```python
from build123d import *

# Parameters (mm, degrees)
SKETCH1_W               = 3.3
SKETCH1_H               = 7.4
BOSS_EXTRUDE1_DEPTH     = 2.6
BOSS_EXTRUDE1_2_DEPTH   = 2.6
BOSS_EXTRUDE1_3_DEPTH   = 2.6
SKETCH1_W_2             = 18
SKETCH1_H_2             = 1.6
BOSS_EXTRUDE1_4_DEPTH   = 2.6
BOSS_EXTRUDE1_5_DEPTH   = 2.6
SKETCH3_W               = 18
SKETCH3_H               = 22.9
BOSS_EXTRUDE2_DEPTH     = 1.6
CUT_EXTRUDE1_DEPTH      = 27.511924597
CUT_EXTRUDE1_DEPTH_BACK = 27.511924597
FILLET1_R               = 2
FILLET2_R               = 1


with BuildPart() as part:
    # Sketch1 → Boss-Extrude1 (new body)
    with BuildSketch(Plane.XY):
        with Locations((-6.907290918, -7.556371191)):
            Rectangle(SKETCH1_W, SKETCH1_H)
    extrude(amount=BOSS_EXTRUDE1_DEPTH)



with BuildPart() as body_2:
    # Sketch1 → Boss-Extrude1 2 (new body)
    with BuildSketch(Plane.XY):
        with Locations((0.442709082, -7.556371191)):
            Rectangle(SKETCH1_W, SKETCH1_H)
    extrude(amount=BOSS_EXTRUDE1_2_DEPTH)


with BuildPart() as body_3:
    # Sketch1 → Boss-Extrude1 3 (new body)
    with BuildSketch(Plane.XY):
        with Locations((7.792709082, -7.556371191)):
            Rectangle(SKETCH1_W, SKETCH1_H)
    extrude(amount=BOSS_EXTRUDE1_3_DEPTH)


with BuildPart() as body_4:
    # Sketch1 → Boss-Extrude1 4 (new body)
    with BuildSketch(Plane.XY):
        with Locations((0.442709082, 3.093628809)):
            Rectangle(SKETCH1_W_2, SKETCH1_H_2)
    extrude(amount=BOSS_EXTRUDE1_4_DEPTH)


with BuildPart() as body_5:
    # Sketch1 → Boss-Extrude1 5 (new body)
    with BuildSketch(Plane.XY):
        with Locations((0.442709082, -18.206371191)):
            Rectangle(SKETCH1_W_2, SKETCH1_H_2)
    extrude(amount=BOSS_EXTRUDE1_5_DEPTH)


with BuildPart() as part_1:
    add(part.part)

    add(body_2.part)  # Boss-Extrude2 merges body 2

    add(body_3.part)  # Boss-Extrude2 merges body 3

    add(body_4.part)  # Boss-Extrude2 merges body 4

    add(body_5.part)  # Boss-Extrude2 merges body 5
    # Sketch3 → Boss-Extrude2 (add)
    with BuildSketch(Plane.XY.offset(2.6)):
        with Locations((0.442709082, -7.556371191)):
            Rectangle(SKETCH3_W, SKETCH3_H)
    extrude(amount=BOSS_EXTRUDE2_DEPTH)

    # Sketch4 → Cut-Extrude1 (cut, two sides: drawn at the far end of the back side and taken through both)
    with BuildSketch(Plane.ZY.offset(8.557290918).offset(-CUT_EXTRUDE1_DEPTH_BACK)):
        Polygon((1.342435563, -8.644254243), (0.613371363, -8.644254243), (0.977903463, -9.008786343), align=None)
        Polygon((2.430318615, -7.556371191), (1.342435563, -6.468488139), (1.342435563, -8.644254243), align=None)
        Polygon((0.977903463, -6.103956039), (0.613371363, -6.468488139), (1.342435563, -6.468488139), align=None)
        Polygon((0.613371363, -6.468488139), (0, -7.081859502), (0, -8.03088288), (0.613371363, -8.644254243), (1.342435563, -8.644254243), (1.342435563, -6.468488139), align=None)
        Polygon((0, -6.468488139), (0, -7.081859502), (0.613371363, -6.468488139), align=None)
        Polygon((0.613371363, -8.644254243), (0, -8.03088288), (0, -8.644254243), align=None)
    extrude(amount=CUT_EXTRUDE1_DEPTH + CUT_EXTRUDE1_DEPTH_BACK, mode=Mode.SUBTRACT)

    # Fillet1
    fillet1_edges = [part_1.edges().sort_by_distance(p)[0] for p in [
        (-8.557290918, 3.893628809, 2.1),
        (9.442709082, 3.893628809, 2.1),
        (9.442709082, -19.006371191, 2.1),
        (-8.557290918, -19.006371191, 2.1),
    ]]
    fillet(fillet1_edges, radius=FILLET1_R)

    # Fillet2
    fillet2_edges = [part_1.edges().sort_by_distance(p)[0] for p in [
        (-8.557290918, -7.556371191, 4.2),
        (0.442709082, 3.893628809, 4.2),
        (0.442709082, -19.006371191, 4.2),
        (9.442709082, -7.556371191, 4.2),
        (-7.97150448, -18.420584754, 4.2),
        (8.856922645, -18.420584754, 4.2),
        (8.856922645, 3.307842371, 4.2),
        (-7.97150448, 3.307842371, 4.2),
    ]]
    fillet(fillet2_edges, radius=FILLET2_R)


solid = part_1.part
```
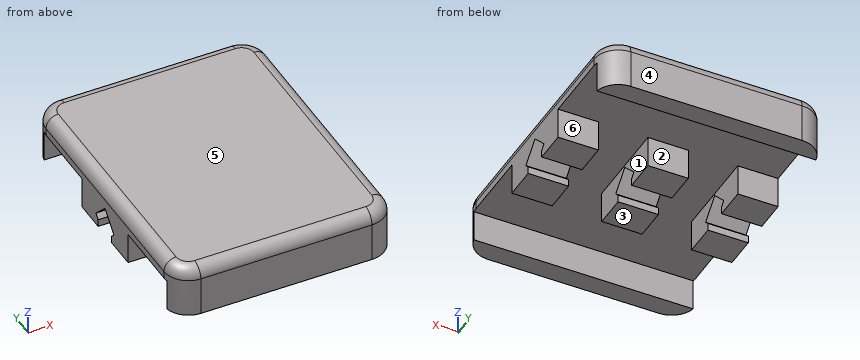
Geometry: final body of the model. Coordinates: model frame, mm. Face numbers are marked on the shaded views. A direction names the side the tool comes from. Round coordinates to 2 decimals unless told otherwise and drop trailing zeros. Loops run counter-clockwise (first coordinate to the right, second up) from the corner with the lowest first, then second, coordinate; pieces in that order, holes last. Notation, with made-up numbers: (-15, -35.5) -> (23, -35.5) arc R23 ccw to (23, -2.5) -> close; hole circle Ø5 at (77.5, -24). An arc over 180 degrees is marked (long way). Use one line per item in the form item = value.
Item 1: Contact query for flat-ended pins moving along their axis: pin 1 Ø1.3 at (x, z) = (8.5, 1) entering from +Y; pin 2 Ø0.7 at (x, z) = (8, 0.5) entering from -Y. Output: stop coordinate, or through.
Evaluation:
pin_1 = 3.85
pin_2 = -19
Item 2: Cut plane A-A on x = -5.5. Output: boundary loops of the cut face in (y, z), then the cut area to 3 significant figures.
Evaluation:
outline = (-19.01, 0) -> (-17.41, 0) -> (-17.41, 2.6) -> (-11.26, 2.6) -> (-11.26, 0) -> (-8.64, 0) -> (-8.64, 0.61) -> (-9.01, 0.98) -> (-7.56, 2.43) -> (-6.1, 0.98) -> (-6.47, 0.61) -> (-6.47, 0) -> (-3.86, 0) -> (-3.86, 2.6) -> (2.29, 2.6) -> (2.29, 0) -> (3.89, 0) -> (3.89, 3.2) arc R1 ccw to (2.89, 4.2) -> (-18.01, 4.2) arc R1 ccw to (-19.01, 3.2) -> close
area = 59.4 mm2
Item 3: Cut plane B-B on y = -11. Output: boundary loops of the cut face in (x, z), then the cut area to 3 significant figures.
Evaluation:
outline = (-8.56, 0) -> (-5.26, 0) -> (-5.26, 2.6) -> (-1.21, 2.6) -> (-1.21, 0) -> (2.09, 0) -> (2.09, 2.6) -> (6.14, 2.6) -> (6.14, 0) -> (9.44, 0) -> (9.44, 3.2) arc R1 ccw to (8.44, 4.2) -> (-7.56, 4.2) arc R1 ccw to (-8.56, 3.2) -> close
area = 54.1 mm2
Item 4: Cut plane C-C on z = 1.5. Give the number of separate pieces and of enclosed holes in the cut face, then the cut area to 3 significant figures.
Evaluation:
separate_pieces = 8
enclosed_holes = 0
area = 109 mm2
Item 5: Access query for the marked faces 1, 2 and 3. Directions: +Z, -Z, +X, -X, +Y, -Y. A direction counts if a zero-diameter tool reaches every point of the face in a straight line with its end or side. Return the directions, or none.
Evaluation:
face_1 = -Z
face_2 = -Z, +X, -X
face_3 = -Z, +X, -X, +Y, -Y
Item 6: Material intervals for probe 1 along X at (y, z) = (-8.25, 1.9); probe 2 along Y at (x, z) = (6.75, 0.4); probe 3 along Y at (x, z) = (-0.5, 2.5), sorted ascending.
Evaluation:
probe_1 = -8.56 to -5.26, -1.21 to 2.09, 6.14 to 9.44
probe_2 = -19.01 to -17.41, -11.26 to -8.64, -6.47 to -3.86, 2.29 to 3.89
probe_3 = -19.01 to -17.41, -11.26 to -3.86, 2.29 to 3.89
Item 7: Cut plane D-D on x = -3. Output: boundary loops of the cut face in (y, z), then the cut area to 3 significant figures.
Evaluation:
outline = (-19.01, 0) -> (-17.41, 0) -> (-17.41, 2.6) -> (2.29, 2.6) -> (2.29, 0) -> (3.89, 0) -> (3.89, 3.2) arc R1 ccw to (2.89, 4.2) -> (-18.01, 4.2) arc R1 ccw to (-19.01, 3.2) -> close
area = 44.5 mm2
Item 8: Draft query along Y for the marked faces 4, 5 and 6. Return one class per face: released by +Y, released by -Y, zero draft, split by the parting line, or undercut.
Evaluation:
face_4 = released by +Y
face_5 = zero draft
face_6 = undercut
